Answer from the drawing. Dimensions are ordinates in mm from the lowest x, y and z of the part. A direction names the side the tool comes from. Coordinates: 2 decimals unless noted, no trailing zeros. Write each loop counter-clockwise with the first axis right and the second up, starting at its lowest first coordinate (ties: lowest second). Pieces come first, ordered by that corner, then holes. Notation, with made-up numbers: (-26, -31.5) -> (-3, -31.5) arc R34 ccw to (-3, 7.5) -> close; hole circle Ø2 at (23, -5.5). An arc over 180 degrees is marked (long way). Answer as a JSON object with one key per item and string values. Group by question number.
(1) Find section B-B (z = 21). Give the vertices of the cut face in (x, y).
(2) For a pull along X with two mould halves and no side action, classify the marked faces 1, 2 and 3 as +X half, -X half, draft (parallel to the pull), parting line (faces both ways), or undercut.
(3) Flat-ended cylindrical pins translate along their axes: P1, Ø5, axis at x = 143.5, z = 78, coming from the -Y side; P2, Ø1, axis at x = 70, z = 76.5, coming from the +Y side; P3, Ø1, axis at y = 74, z = 36.5, coming from the -X side. Find the tip coordinate at first contact, or state that the pin passes through.
(4) Find section A-A (y = 101). Give the vertices of the cut face in (x, z), then the cut area to 3 significant figures.
(5) Which of the six approach directions +Z, -Z, +X, -X, +Y, -Y give full straight-line access (tool end or side, diameter ignored) to the marked faces 4 and 5?
(6) Straight lines are drawn through the part: L1, parallel to X at y = 144.5, z = 84; L2, parallel to Y at x = 148, z = 65.5; L3, parallel to X at y = 85.5, z = 65.5. For each, find the intervals that lie inside material, in ascending order.
(7) Find section C-C (x = 148.5). Give the vertices of the cut face in (y, z), then the cut area to 3 significant figures.
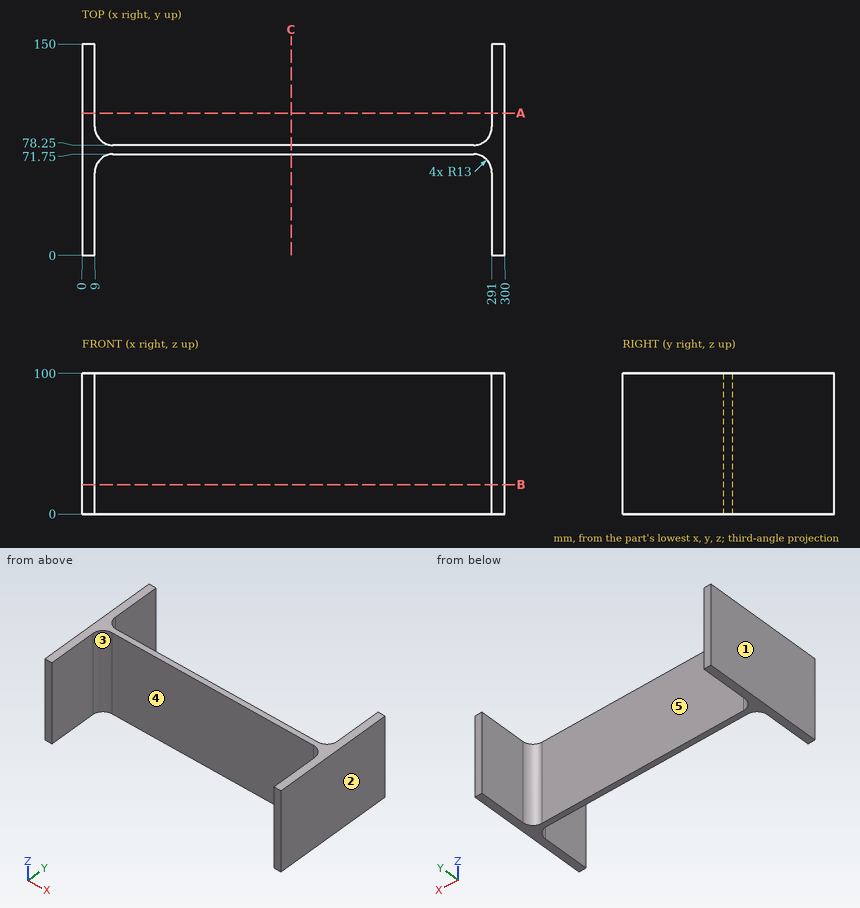
Results below:
{
 "1": {"outline": "(0, 0) -> (9, 0) -> (9, 58.75) arc R13 cw to (22, 71.75) -> (278, 71.75) arc R13 cw to (291, 58.75) -> (291, 0) -> (300, 0) -> (300, 150) -> (291, 150) -> (291, 91.25) arc R13 cw to (278, 78.25) -> (22, 78.25) arc R13 cw to (9, 91.25) -> (9, 150) -> (0, 150) -> close"},
 "2": {"face 1": "-X half", "face 2": "+X half", "face 3": "undercut"},
 "3": {"P1": "stops at y = 71.75", "P2": "stops at y = 78.25", "P3": "stops at x = 0"},
 "4": {"outline": "(0, 0) -> (9, 0) -> (9, 100) -> (0, 100) -> close; (291, 0) -> (300, 0) -> (300, 100) -> (291, 100) -> close", "area": "1,800 mm2"},
 "5": {"face 4": "+Z, -Z, -Y", "face 5": "+Z, -Z, +Y"},
 "6": {"L1": "x = 0 to 9, 291 to 300", "L2": "y = 71.75 to 78.25", "L3": "x = 0 to 10.34, 289.66 to 300"},
 "7": {"outline": "(71.75, 0) -> (78.25, 0) -> (78.25, 100) -> (71.75, 100) -> close", "area": "650 mm2"}
}
